Autodesk Inventor part; units mm, degrees
ref_plane "YZ Plane" through (0, 0, 0) normal (1, 0, 0) x (0, 1, 0)
ref_plane "XZ Plane" through (0, 0, 0) normal (0, 1, 0) x (-1, 0, 0)
ref_plane "XY Plane" through (0, 0, 0) normal (0, 0, 1) x (1, 0, 0)
sketch "Sketch1" plane through (0, 0, 0) normal (0, 0, 1) x (1, 0, 0)
  circle A0 centre (0, 0) radius 38.1
  dimension "d0" = 76.2
extrude "Extrusion1" add sketch "Sketch1" along normal blind 2.54
sketch "Sketch5" plane through (0, 0, 2.54) normal (0, 0, 1) x (1, 0, 0)
  circle A0 centre (0, 0) radius 15.24
  dimension "d24" = 30.48
extrude "Extrusion7" add sketch "Sketch5" along normal blind 2.54
sketch "Sketch6" plane through (0, 0, 5.08) normal (0, 0, 1) x (1, 0, 0)
  line L0 (0, 0) -> (0, 10.9985)
  circle A0 centre (0, 10.9985) radius 1.27
  circle A1 centre (-9.525, -5.4993) radius 1.27
  circle A2 centre (9.525, -5.4993) radius 1.27
  dimension "d28" = 2.54
  dimension "d31" = 360
  dimension "d49" = 19.05
extrude "Extrusion8" cut sketch "Sketch6" against normal through all
sketch "Sketch7" plane through (0, 0, 5.08) normal (0, 0, 1) x (1, 0, 0)
  circle A0 centre (0, 0) radius 3.175
  dimension "d35" = 6.35
extrude "Extrusion9" cut sketch "Sketch7" against normal blind 3.175
sketch "Sketch8" plane through (0, 0, 1.905) normal (0, 0, 1) x (1, 0, 0)
  circle A0 centre (0, 0) radius 2.3812
  dimension "d38" = 4.7625
extrude "Extrusion10" cut sketch "Sketch8" against normal through all
sketch "Sketch9" plane through (0, 0, 2.54) normal (0, 0, 1) x (1, 0, 0)
  line L0 (0, 0) -> (0, 30.48)
  circle A0 centre (0, 30.48) radius 1.5875
  circle A1 centre (-26.3965, 15.24) radius 1.5875
  circle A2 centre (-26.3965, -15.24) radius 1.5875
  circle A3 centre (0, -30.48) radius 1.5875
  circle A4 centre (26.3965, -15.24) radius 1.5875
  circle A5 centre (26.3965, 15.24) radius 1.5875
  dimension "d41" = 30.48
  dimension "d42" = 3.175
  dimension "d45" = 360
extrude "Extrusion11" cut sketch "Sketch9" against normal blind 25.4
chamfer "Chamfer1" distance 2.667 distance2 1.27 1 edges at (-15.24, 0, 5.08) measured on face at (4.9695, 7.5399, 5.08)
properties part number "SpoolEndSpurSideLargeSpur" material "ABS Plastic"
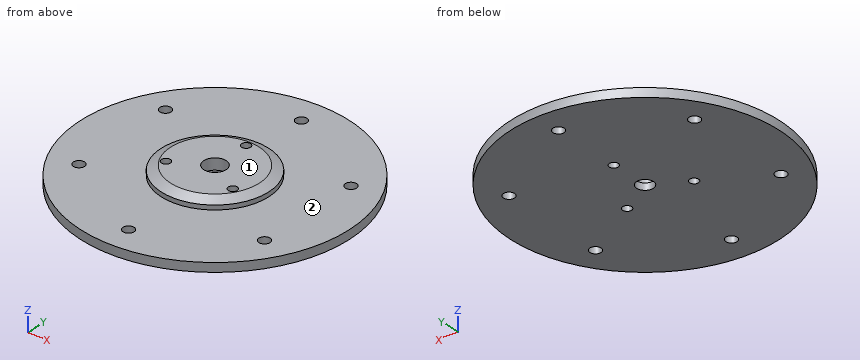
The model under review builds one solid part; all positions refer to its coordinate system, in mm. Face numbers are marked on the shaded views. A direction names the side the tool comes from. Round coordinates to 2 decimals unless told otherwise and drop trailing zeros. Order: outer loops, then holes, each group sorted by start corner. A loop starts at its lowest first (then second) coordinate and runs counter-clockwise, first axis right, second up.
(1) Wall thickness on L1, parallel to Y at x = 0, z = 2.05 (1 decimal); L2, parallel to Y at x = 0, z = 1; L3, parallel to Y at x = 0, z = 3.55 (1 decimal): over which ranges is each line inside the solid? List them lowest first.
Working result:
L1: y = -38.1 to -32.1, -28.9 to -3.2, 3.2 to 9.7, 12.3 to 28.9, 32.1 to 38.1
L2: y = -38.1 to -32.07, -28.89 to -2.38, 2.38 to 9.73, 12.27 to 28.89, 32.07 to 38.1
L3: y = -15.2 to -3.2, 3.2 to 9.7, 12.3 to 15.2
(2) Take a section at B-B, the plane y = 30.48. State the section outline as (x, z) points.
Working result:
outline: (-22.86, 0) - (-1.59, 0) - (-1.59, 2.54) - (-22.86, 2.54) - close; (1.59, 0) - (22.86, 0) - (22.86, 2.54) - (1.59, 2.54) - close
(3) Tool access review of the marked faces 1 and 2: name each direction out of +Z, -Z, +X, -X, +Y, -Y from which nothing blocks a thin tool from reaching the whole face with its end or side.
Working result:
face 1: +Z, +X, -X, +Y, -Y
face 2: +Z
(4) For P1, Ø3, axis at x = 0, y = -30.48, coming from the +Z side; P2, Ø3.5, axis at x = 0, y = 30.48, coming from the +Z side; P3, Ø3, axis at x = -1.5, y = 0, coming from the +Z side (3 decimals), all flat-tipped, find the tip position at first contact; note any pin that passes through.
Working result:
P1: passes through
P2: stops at z = 2.54
P3: stops at z = 1.905
(5) Take a section at A-A, the plane x = 0. Count the separate pieces of the cut face and the enclosed holes in it, plus the area to 3 significant figures.
Working result:
separate pieces: 5
enclosed holes: 0
area: 209 mm2
(6) Take a section at C-C, the plane x = -21. State the section outline as (y, z) points, plus the area to 3 significant figures.
Working result:
outline: (-31.79, 0) - (31.79, 0) - (31.79, 2.54) - (-31.79, 2.54) - close
area: 161 mm2
(7) Take a section at D-D, the plane x = -33. State the section outline as (y, z) points, plus the area to 3 significant figures.
Working result:
outline: (-19.04, 0) - (19.04, 0) - (19.04, 2.54) - (-19.04, 2.54) - close
area: 96.7 mm2
